Geometry check sheet. Reference: the model listing, model coordinates, mm. A direction names the side the tool comes from. Give positions to 0.01 mm unless a question says otherwise; leave off trailing zeros. Loops run counter-clockwise (first coordinate to the right, second up) from the corner with the lowest first, then second, coordinate; pieces in that order, holes last. Notation, with made-up numbers: (-16.75, 42.5) -> (-0.75, 42.5) arc R29 ccw to (-0.75, 70.5) -> close; hole circle Ø2 at (-5, -37.5). An arc over 180 degrees is marked (long way). One line per question, with ' | ' between items.
from build123d import *

# Parameters (mm, degrees)
BOSS_EXTRUDE1_DEPTH      = 469.9
SKETCH2_W                = 10.16
SKETCH2_H                = 83.810703233
SKETCH2_H_2              = 111.159792755
SKETCH2_H_3              = 83.757510526
SKETCH2_H_4              = 83.784106879
SKETCH2_H_5              = 83.730914172
SKETCH2_H_6              = 83.704317819
SKETCH2_H_7              = 83.677721465
SKETCH2_H_8              = 83.651125112
SKETCH2_H_9              = 22.104476438
CUT_EXTRUDE1_DEPTH       = 10.16
SKETCH3_W                = 10.16
SKETCH3_H                = 55.879999965
SKETCH3_H_2              = 88.9
SKETCH3_H_3              = 109.22
CUT_EXTRUDE2_DEPTH       = 12.7
SKETCH4_W                = 84.113540858
SKETCH4_H                = 20.32
CUT_EXTRUDE3_DEPTH       = 12.7
SKETCH5_W                = 89.916
SKETCH5_H                = 20.32
CUT_EXTRUDE4_DEPTH       = 12.7
SKETCH13_R               = 3.175
CUT_EXTRUDE8_DEPTH       = 2128.667464702
CUT_EXTRUDE9_DEPTH       = 2128.667464702
SKETCH20_R               = 4.7625
CUT_EXTRUDE10_DEPTH      = 2107.728843747
SKETCH24_R               = 3.175
CUT_EXTRUDE12_DEPTH      = 12.7
CUT_EXTRUDE13_DEPTH      = 2128.667464702
CUT_EXTRUDE13_DEPTH_BACK = 2128.667464702


with BuildPart() as part:
    # Sketch1 → Boss-Extrude1 (new body)
    with BuildSketch(Plane.XY):
        Polygon((-215.881789204, 2052.32), (-215.881789204, 1463.040000035), (-316.088635901, 20.32), (-317.499999939, 0), (-307.333509538, 0), (-205.715298803, 1463.040000035), (-205.715298803, 2072.64), (-215.881789204, 2072.64), align=None)
    extrude(amount=-BOSS_EXTRUDE1_DEPTH)

    # Sketch2 → Cut-Extrude1 (cut)
    with BuildSketch(Plane(origin=(-315.975651309, 21.946686571, 0), x_dir=(0, 0, 1), z_dir=(-0.9975965627192115, 0.06928995634877068, 0))):
        with Locations((-5.08, 247.132760087)):
            Rectangle(SKETCH2_W, SKETCH2_H)
        with Locations((-5.08, 55.684811679)):
            Rectangle(SKETCH2_W, SKETCH2_H_2)
        with Locations((-5.08, 602.706163733)):
            Rectangle(SKETCH2_W, SKETCH2_H_3)
        with Locations((-5.08, 424.91946191)):
            Rectangle(SKETCH2_W, SKETCH2_H_4)
        with Locations((-5.08, 780.492865556)):
            Rectangle(SKETCH2_W, SKETCH2_H_5)
        with Locations((-5.08, 958.27956738)):
            Rectangle(SKETCH2_W, SKETCH2_H_6)
        with Locations((-5.08, 1136.066269203)):
            Rectangle(SKETCH2_W, SKETCH2_H_7)
        with Locations((-5.08, 1313.852971026)):
            Rectangle(SKETCH2_W, SKETCH2_H_8)
        with Locations((-5.08, -10.947322918)):
            Rectangle(SKETCH2_W, SKETCH2_H_9)
        with Locations((-464.82, -10.947322918)):
            Rectangle(SKETCH2_W, SKETCH2_H_9)
        with Locations((-464.82, 55.684811679)):
            Rectangle(SKETCH2_W, SKETCH2_H_2)
        with Locations((-464.82, 247.132760087)):
            Rectangle(SKETCH2_W, SKETCH2_H)
        with Locations((-464.82, 424.91946191)):
            Rectangle(SKETCH2_W, SKETCH2_H_4)
        with Locations((-464.82, 602.706163733)):
            Rectangle(SKETCH2_W, SKETCH2_H_3)
        with Locations((-464.82, 780.492865556)):
            Rectangle(SKETCH2_W, SKETCH2_H_5)
        with Locations((-464.82, 958.27956738)):
            Rectangle(SKETCH2_W, SKETCH2_H_6)
        with Locations((-464.82, 1136.066269203)):
            Rectangle(SKETCH2_W, SKETCH2_H_7)
        with Locations((-464.82, 1313.852971026)):
            Rectangle(SKETCH2_W, SKETCH2_H_8)
    extrude(amount=-CUT_EXTRUDE1_DEPTH, mode=Mode.SUBTRACT)

    # Sketch3 → Cut-Extrude2 (cut)
    with BuildSketch(Plane.ZY.offset(215.881789204)):
        with Locations((-5.08, 1490.980000018)):
            Rectangle(SKETCH3_W, SKETCH3_H)
        with Locations((-5.08, 1652.27)):
            Rectangle(SKETCH3_W, SKETCH3_H_2)
        Polygon((-469.9, 1463.040000035), (-459.727704291, 1463.040000035), (-455.605912768, 1546.794803777), (-465.753631921, 1547.294199405), (-461.607263841, 1631.548398775), (-451.459544688, 1631.049003148), (-447.313176609, 1715.303202518), (-457.460895762, 1715.802598146), (-453.314527682, 1800.056797516), (-443.166808529, 1799.557401889), (-439.02044045, 1883.811601259), (-449.168159603, 1884.310996887), (-445.021791523, 1968.565196257), (-434.87407237, 1968.06580063), (-429.727704291, 2072.64), (-469.9, 2072.64), align=None)
        with Locations((-5.08, 1830.07)):
            Rectangle(SKETCH3_W, SKETCH3_H_2)
        with Locations((-5.08, 2018.03)):
            Rectangle(SKETCH3_W, SKETCH3_H_3)
    extrude(amount=-CUT_EXTRUDE2_DEPTH, mode=Mode.SUBTRACT)

    # Sketch4 → Cut-Extrude3 (cut)
    with BuildSketch(Plane.ZY.offset(215.881789204)):
        with Locations((-388.670933862, 2062.48)):
            Rectangle(SKETCH4_W, SKETCH4_H)
        with Locations((-220.443852145, 2062.48)):
            Rectangle(SKETCH4_W, SKETCH4_H)
        with Locations((-52.216770429, 2062.48)):
            Rectangle(SKETCH4_W, SKETCH4_H)
    extrude(amount=-CUT_EXTRUDE3_DEPTH, mode=Mode.SUBTRACT)

    # Sketch5 → Cut-Extrude4 (cut)
    with BuildSketch(Plane(origin=(-315.975651309, 21.946686571, 0), x_dir=(0, 0, 1), z_dir=(-0.9975965627192115, 0.06928995634877068, 0))):
        with Locations((-414.782, -11.839561137)):
            Rectangle(SKETCH5_W, SKETCH5_H)
        with Locations((-234.95, -11.839561137)):
            Rectangle(SKETCH5_W, SKETCH5_H)
        with Locations((-55.118, -11.839561137)):
            Rectangle(SKETCH5_W, SKETCH5_H)
    extrude(amount=-CUT_EXTRUDE4_DEPTH, mode=Mode.SUBTRACT)

    # Sketch13 → Cut-Extrude8 (cut, through all)
    with BuildSketch(Plane.ZY.offset(215.881789204)):
        with Locations(Location((-25.246459893, 1731.87, 0), (0, 0, 270))):
            Circle(SKETCH13_R)
        with Locations(Location((-70.408959893, 1755.42, 0), (0, 0, 270))):
            Circle(SKETCH13_R)
        with Locations(Location((-182.408959893, 1755.42, 0), (0, 0, 270))):
            Circle(SKETCH13_R)
        with Locations(Location((-25.246459893, 1918.97, 0), (0, 0, 270))):
            Circle(SKETCH13_R)
        with Locations(Location((-47.788959893, 1865.42, 0), (0, 0, 270))):
            Circle(SKETCH13_R)
        with Locations(Location((-182.408959893, 1910.42, 0), (0, 0, 270))):
            Circle(SKETCH13_R)
        with Locations(Location((-117.078959893, 1910.42, 0), (0, 0, 270))):
            Circle(SKETCH13_R)
        with Locations(Location((-70.408959893, 1895.42, 0), (0, 0, 270))):
            Circle(SKETCH13_R)
        with Locations(Location((-317.028959893, 1865.42, 0), (0, 0, 270))):
            Circle(SKETCH13_R)
        with Locations(Location((-294.408959893, 1755.42, 0), (0, 0, 270))):
            Circle(SKETCH13_R)
        with Locations(Location((-317.028959893, 1785.42, 0), (0, 0, 270))):
            Circle(SKETCH13_R)
        with Locations(Location((-339.571459893, 1731.87, 0), (0, 0, 270))):
            Circle(SKETCH13_R)
        with Locations(Location((-339.571459893, 1918.97, 0), (0, 0, 270))):
            Circle(SKETCH13_R)
    extrude(amount=-CUT_EXTRUDE8_DEPTH, mode=Mode.SUBTRACT)

    # Sketch17 → Cut-Extrude9 (cut, through all)
    with BuildSketch(Plane.ZY.offset(215.881789204)):
        Polygon((-91.602336227, 1471.504269383), (-81.702736369, 1473.789772095), (-94.643375784, 1529.841839519), (-104.542975642, 1527.556336807), align=None)
        Polygon((-130.424254473, 1639.660471655), (-117.483615058, 1583.608404231), (-107.584015199, 1585.893906943), (-120.524654614, 1641.945974367), align=None)
    extrude(amount=-CUT_EXTRUDE9_DEPTH, mode=Mode.SUBTRACT)

    # Sketch20 → Cut-Extrude10 (cut, through all)
    with BuildSketch(Plane(origin=(-315.975651309, 21.946686571, 0), x_dir=(0, 0, 1), z_dir=(-0.9975965627192116, 0.06928995634876853, 0))):
        with Locations(Location((-35.56, 347.287639338, 0), (0, 0, 270))):
            Circle(SKETCH20_R)
        with Locations(Location((-35.56, 302.837639338, 0), (0, 0, 270))):
            Circle(SKETCH20_R)
        Polygon((-120.929306778, 445.712379572), (-154.823537638, 399.698212032), (-162.492565561, 405.347250509), (-128.598334701, 451.361418049), align=None)
    extrude(amount=-CUT_EXTRUDE10_DEPTH, mode=Mode.SUBTRACT)

    # Sketch24 → Cut-Extrude12 (cut)
    with BuildSketch(Plane.ZY.offset(215.881789204)):
        with Locations(Location((-39.313746491, 1670.454214013, 0), (0, 0, 270))):
            Circle(SKETCH24_R)
    extrude(amount=-CUT_EXTRUDE12_DEPTH, mode=Mode.SUBTRACT)

    # Sketch26 → Cut-Extrude13 (cut, two sides: drawn at the far end of the back side and taken through both)
    with BuildSketch(Plane.ZY.offset(215.881789204).offset(-CUT_EXTRUDE13_DEPTH_BACK)):
        Polygon((-117.688081031, 385.528057798), (-109.500847052, 379.511801077), (-55.568463259, 452.553412636), (-63.755697238, 458.569669358), align=None)
        Polygon((-171.620464825, 312.486446238), (-225.552848619, 239.444834679), (-217.372552167, 233.433675887), (-163.440168374, 306.475287447), align=None)
        Polygon((-22.52887933, 606.973028774), (-44.10850301, 653.102617965), (-53.31924736, 648.814478552), (-31.73962368, 602.684889361), align=None)
        Polygon((-74.89887104, 694.944067742), (-65.68812669, 699.232207156), (-87.26775037, 745.361796346), (-96.478494721, 741.073656933), align=None)
        Polygon((-279.485232413, 166.403223119), (-333.417616206, 93.36161156), (-325.230382227, 87.345354838), (-271.297998434, 160.386966398), align=None)
    extrude(amount=CUT_EXTRUDE13_DEPTH + CUT_EXTRUDE13_DEPTH_BACK, mode=Mode.SUBTRACT)


solid = part.part
Item 1: Scan lines: probe 1 along Z at (x, y) = (-207.75, 1918.97); probe 2 along Z at (x, y) = (-209, 1755.42); probe 3 along X at (y, z) = (243, -152). Record each from-to range of solid material in increasing order.
Result:
probe 1: -447.46 to -342.75, -336.4 to -28.42, -22.07 to 0 | probe 2: -455.51 to -297.58, -291.23 to -185.58, -179.23 to -73.58, -67.23 to 0 | probe 3: -300.62 to -290.46
Item 2: Release check for a two-part mould opening along Y. For faces 5 (the face through (-257.236, 721.279, -231.661)), 6 (the face through (-293.56, 269.443, -190.784)), 7 (the face through (-215.882, 1772, -230)) record: pulls with the +Y half, pulls with the -Y half, needs draft (parallel to the pull), parting line crosses it, or undercut.
Result:
face 5: pulls with the -Y half | face 6: undercut | face 7: needs draft
Item 3: Sectioned sample at A-A (z = -392). Record the cut outline in (x, y), plus the area to 3 significant figures.
Result:
outline: (-316.09, 20.27) -> (-305.97, 19.57) -> (-205.72, 1463.04) -> (-205.72, 2052.32) -> (-215.88, 2052.32) -> (-215.88, 1463.04) -> close | area: 20,700 mm2
Item 4: Depth check by flat-ended pin: pin 1 Ø3 at (x, z) = (-210.5, -7.5) entering from -Y; pin 2 Ø5 at (x, y) = (-222.5, 1348) entering from -Z; pin 3 Ø1 at (y, z) = (970.5, -145.5) entering from +X; pin 4 Ø4 at (y, z) = (1755.42, -70.41) entering from -X. Enter the tip coordinate at first touch or a pass-through.
Result:
pin 1: y = 1373.66 | pin 2: z = -459.74 | pin 3: x = -239.89 | pin 4: through
Item 5: Sectioned sample at B-B (y = 1081.5). Record the cut outline in (x, z).
Result:
outline: (-242.38, -469.9) -> (-232.22, -469.9) -> (-232.22, 0) -> (-242.38, 0) -> close
Item 6: Set-up check for faces 1 (the face through (-281.329, 448.604, -145.783)), 2 (the face through (-205.715, 1764, -230)), 3 (the face through (-281.68, 443.61, -137.64)), 4 (the face through (-303.289, 130.394, -306.074)): record each of +Z, -Z, +X, -X, +Y, -Y from which the full face is reachable in a straight line by a thin tool's end or side.
Result:
face 1: -X | face 2: +Z, -Z, +X, +Y, -Y | face 3: +X | face 4: +X, -X
